```python
from build123d import *

# Parameters (mm, degrees)
SKETCH_1_R      = 1.25
SKETCH_1_R_2    = 1
EXTRUDE_1_DEPTH = 2


with BuildPart() as part:
    # 草圖1 → 填料-伸長1 (new body)
    with BuildSketch(Plane.XY):
        with BuildLine():
            Line((25.714690816, 4.04468624), (25.714690816, -0.95531376))
            Line((25.714690816, -0.95531376), (25.714690816, -12.45531376))
            ThreePointArc((25.714690816, -12.45531376), (25.421797597, -13.162420542), (24.714690816, -13.45531376))
            Line((24.714690816, -13.45531376), (-14.285309184, -13.45531376))
            ThreePointArc((-14.285309184, -13.45531376), (-14.992415965, -13.162420542), (-15.285309184, -12.45531376))
            Line((-15.285309184, -12.45531376), (-15.285309184, 3.54468624))
            ThreePointArc((-15.285309184, 3.54468624), (-14.285309184, 4.54468624), (-15.285309184, 5.54468624))
            Line((-15.285309184, 5.54468624), (-17.285309184, 5.54468624))
            Line((-17.285309184, 5.54468624), (-17.285309184, 9.54468624))
            Line((-17.285309184, 9.54468624), (-15.285309184, 9.54468624))
            ThreePointArc((-15.285309184, 9.54468624), (-14.285309184, 10.54468624), (-15.285309184, 11.54468624))
            Line((-15.285309184, 11.54468624), (-15.285309184, 15.54468624))
            ThreePointArc((-15.285309184, 15.54468624), (-14.285309184, 16.54468624), (-15.285309184, 17.54468624))
            Line((-15.285309184, 17.54468624), (-17.285309184, 17.54468624))
            Line((-17.285309184, 17.54468624), (-17.285309184, 21.54468624))
            Line((-17.285309184, 21.54468624), (-15.285309184, 21.54468624))
            ThreePointArc((-15.285309184, 21.54468624), (-14.285309184, 22.54468624), (-15.285309184, 23.54468624))
            Line((-15.285309184, 23.54468624), (-15.285309184, 39.54468624))
            ThreePointArc((-15.285309184, 39.54468624), (-14.992415965, 40.251793021), (-14.285309184, 40.54468624))
            Line((-14.285309184, 40.54468624), (24.714690816, 40.54468624))
            ThreePointArc((24.714690816, 40.54468624), (25.421797597, 40.251793021), (25.714690816, 39.54468624))
            Line((25.714690816, 39.54468624), (25.714690816, 28.54468624))
            Line((25.714690816, 28.54468624), (25.714690816, 23.04468624))
            ThreePointArc((25.714690816, 23.04468624), (25.421797597, 22.337579458), (24.714690816, 22.04468624))
            Line((24.714690816, 22.04468624), (20.714690816, 22.04468624))
            ThreePointArc((20.714690816, 22.04468624), (20.007584035, 21.751793021), (19.714690816, 21.04468624))
            Line((19.714690816, 21.04468624), (19.714690816, 6.04468624))
            ThreePointArc((19.714690816, 6.04468624), (20.007584035, 5.337579458), (20.714690816, 5.04468624))
            Line((20.714690816, 5.04468624), (24.714690816, 5.04468624))
            ThreePointArc((24.714690816, 5.04468624), (25.421797597, 4.751793021), (25.714690816, 4.04468624))
        make_face()
        with Locations((-6.785309184, 27.04468624)):
            Circle(SKETCH_1_R, mode=Mode.SUBTRACT)
        with Locations((23.214690816, 27.04468624)):
            Circle(SKETCH_1_R, mode=Mode.SUBTRACT)
        with Locations((-6.785309184, 0.04468624)):
            Circle(SKETCH_1_R, mode=Mode.SUBTRACT)
        with Locations((23.214690816, 0.04468624)):
            Circle(SKETCH_1_R, mode=Mode.SUBTRACT)
        with Locations((-12.785309184, 33.04468624)):
            Circle(SKETCH_1_R, mode=Mode.SUBTRACT)
        with Locations((23.214690816, 33.04468624)):
            Circle(SKETCH_1_R, mode=Mode.SUBTRACT)
        with Locations(Location((23.214690816, -5.95531376, 0), (0, 0, 180))):
            Circle(SKETCH_1_R, mode=Mode.SUBTRACT)
        with Locations(Location((-12.785309184, -5.95531376, 0), (0, 0, 180))):
            Circle(SKETCH_1_R, mode=Mode.SUBTRACT)
        with Locations((-13.285309184, 19.54468624)):
            Circle(SKETCH_1_R_2, mode=Mode.SUBTRACT)
        with Locations((-13.285309184, 7.54468624)):
            Circle(SKETCH_1_R_2, mode=Mode.SUBTRACT)
        with BuildLine():
            Line((3.214690816, 22.04468624), (8.214690816, 22.04468624))
            ThreePointArc((8.214690816, 22.04468624), (11.750224722, 20.580220146), (13.214690816, 17.04468624))
            Line((13.214690816, 17.04468624), (13.214690816, 10.04468624))
            ThreePointArc((13.214690816, 10.04468624), (11.750224722, 6.509152334), (8.214690816, 5.04468624))
            Line((8.214690816, 5.04468624), (3.214690816, 5.04468624))
            ThreePointArc((3.214690816, 5.04468624), (-0.32084309, 6.509152334), (-1.785309184, 10.04468624))
            Line((-1.785309184, 10.04468624), (-1.785309184, 17.04468624))
            ThreePointArc((-1.785309184, 17.04468624), (-0.32084309, 20.580220146), (3.214690816, 22.04468624))
        make_face(mode=Mode.SUBTRACT)
    extrude(amount=EXTRUDE_1_DEPTH)


solid = part.part
```
Input: part model. Units: mm. Frame: model coordinates. A direction names the side the tool comes from. Round coordinates to 2 decimals unless told otherwise and drop trailing zeros. Write each loop counter-clockwise with the first axis right and the second up, starting at its lowest first coordinate (ties: lowest second). Pieces come first, ordered by that corner, then holes. Notation, with made-up numbers: (70, -10.75) -> (111, -10.75) arc R17 ccw to (111, -4.75) -> close; hole circle Ø9 at (86.5, 89.25). An arc over 180 degrees is marked (long way). Answer as CSV lines item,"result".
1. Section B-B (x = 23). Return the cut outline in (y, z).
Geometry says:
outline,"(-13.46, 0) -> (-7.19, 0) -> (-7.19, 2) -> (-13.46, 2) -> close; (-4.72, 0) -> (-1.19, 0) -> (-1.19, 2) -> (-4.72, 2) -> close; (1.28, 0) -> (5.04, 0) -> (5.04, 2) -> (1.28, 2) -> close; (22.04, 0) -> (25.81, 0) -> (25.81, 2) -> (22.04, 2) -> close; (28.28, 0) -> (31.81, 0) -> (31.81, 2) -> (28.28, 2) -> close; (34.28, 0) -> (40.54, 0) -> (40.54, 2) -> (34.28, 2) -> close"
2. Section A-A (x = 9). Return the cut outline in (y, z).
Geometry says:
outline,"(-13.46, 0) -> (5.11, 0) -> (5.11, 2) -> (-13.46, 2) -> close; (21.98, 0) -> (40.54, 0) -> (40.54, 2) -> (21.98, 2) -> close"
3. Reachability of faces 4 (the cylindrical face through (11.79, 6.55, 0.99)), 5 (the flat face through (23, 5.045, 1)), 6 (the flat face through (-15.285, -5, 1)) from +Z, -Z, +X, -X, +Y, -Y: full face, straight path, thin tool, end or side. Return the list, or none.
Geometry says:
face 4,"+Z, -Z"
face 5,"+Z, -Z, +X"
face 6,"+Z, -Z, -X, -Y"
4. Mould query, pull axis X, two halves, no side actions, for faces 1 (the cylindrical face through (-14.286, 22.523, 0.986)), 2 (the cylindrical face through (-7.056, 25.824, 0.986)), 3 (the flat face through (5, 40.545, 1)). Classes: +X half, -X half, draft (parallel to the pull), parting line (faces both ways), or undercut.
Geometry says:
face 1,"-X half"
face 2,"undercut"
face 3,"draft"
5. Ray query, L1, parallel to X at y = 0, z = 1.4; L2, parallel to Y at x = 23.5, z = 1.65; L3, parallel to Y at x = 8.5, z = 1.65. Return the intervals inside material, ascending. Write a range as [from, to].
Geometry says:
L1,"x = [-15.29, -8.03], [-5.54, 21.97], [24.46, 25.71]"
L2,"y = [-13.46, -7.17], [-4.74, -1.17], [1.26, 5.04], [22.04, 25.83], [28.26, 31.83], [34.26, 40.54]"
L3,"y = [-13.46, 5.05], [22.04, 40.54]"
6. Section D-D (x = -6.5). Return the cut outline in (y, z), plus the area to 3 significant figures.
Geometry says:
outline,"(-13.46, 0) -> (-1.17, 0) -> (-1.17, 2) -> (-13.46, 2) -> close; (1.26, 0) -> (25.83, 0) -> (25.83, 2) -> (1.26, 2) -> close; (28.26, 0) -> (40.54, 0) -> (40.54, 2) -> (28.26, 2) -> close"
area,"98.3 mm^2"
7. Section C-C (y = -3.5). Return the cut outline in (x, z), plus the area to 3 significant figures.
Geometry says:
outline,"(-15.29, 0) -> (25.71, 0) -> (25.71, 2) -> (-15.29, 2) -> close"
area,"82.0 mm^2"
8. Contact query for flat-ended pins moving along their axis: P1, Ø0.6, axis at x = -16, z = 1, coming from the +Y side; P2, Ø1, axis at x = -16.5, z = 1, coming from the -Y side; P3, Ø0.6, axis at y = 13.5, z = 0.5, coming from the -X side; P4, Ø3, axis at x = -6.79, y = 0.04, coming from the -Z side. Output: stop coordinate, or through.
Geometry says:
P1,"stops at y = 21.54"
P2,"stops at y = 5.54"
P3,"stops at x = -15.29"
P4,"stops at z = 0"
